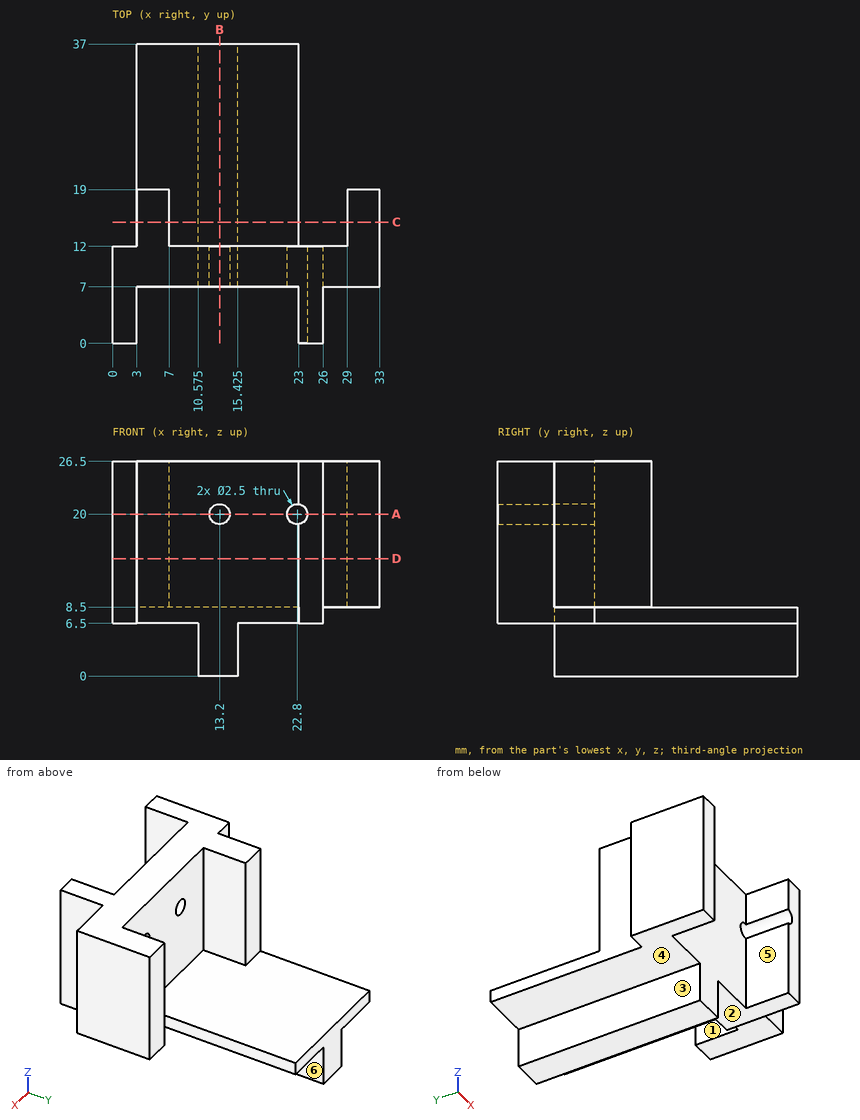
The drawing under review shows one solid part. Ordinate dimensions are in mm from its lowest x, y, z. A direction names the side the tool comes from. Coordinates: 2 decimals unless noted, no trailing zeros. Order: outer loops, then holes, each group sorted by start corner. A loop starts at its lowest first (then second) coordinate and runs counter-clockwise, first axis right, second up. Notation, with made-up numbers: (4, 5.25) -> (31, 5.25) arc R21 ccw to (31, 18.25) -> close; hole circle Ø10 at (-10, -31). An arc over 180 degrees is marked (long way). Answer in a Markdown table with one row per item. Add a question column.
Item 1: We need section B-B on x = 13.2. Write out the cut boundary in (y, z), plus the area to 4 significant figures.
Item 2: We need section D-D on z = 14.5. Write out the cut boundary in (x, y).
Item 3: Mouldability with a two-part tool opening along X and no side actions: class the marked faces 4, 5 and 6 as +X half, -X half, draft (parallel to the pull), parting line (faces both ways), or undercut.
Item 4: Clearance check with flat-ended pins moving along their axes: pin 1 (3 mm diameter, centred on x = 13.2, z = 20, fed in from -Y); pin 2 (3 mm diameter, centred on x = 7.5, y = 14, fed in from -Z); pin 3 (3 mm diameter, centred on x = 30.5, z = 17, fed in from +Y). State where each tip first meets the part, or that it passes through.
Item 5: To check wall thickness, follow probe 1 along X at (y, z) = (8.5, 20); probe 2 along X at (y, z) = (13.5, 24.5); probe 3 along X at (y, z) = (3.5, 16.75). State the ranges of each line that lie inside material, in increasing order.
Item 6: We need section A-A on z = 20. Write out the cut boundary in (x, y).
Item 7: We need section C-C on y = 15. Write out the cut boundary in (x, z) (3 decimals).
Item 8: Machinability: for the marked faces 1, 2 and 3, which of the approach directions +Z, -Z, +X, -X, +Y, -Y give a long, thin tool a straight path to every point of the face, cutting with its end or side? Answer none if there is none.
Final values:
| question | item | result |
|---|---|---|
| 1 | outline | (7, 0) -> (37, 0) -> (37, 8.5) -> (12, 8.5) -> (12, 18.75) -> (7, 18.75) -> close; (7, 21.25) -> (12, 21.25) -> (12, 26.5) -> (7, 26.5) -> close |
| 1 | area | 332.5 mm2 |
| 2 | outline | (0, 0) -> (3, 0) -> (3, 7) -> (23, 7) -> (23, 0) -> (26, 0) -> (26, 7) -> (33, 7) -> (33, 19) -> (29, 19) -> (29, 12) -> (7, 12) -> (7, 19) -> (3, 19) -> (3, 12) -> (0, 12) -> close |
| 3 | face 4 | draft |
| 3 | face 5 | undercut |
| 3 | face 6 | +X half |
| 4 | pin 1 | stops at y = 7 |
| 4 | pin 2 | stops at z = 6.5 |
| 4 | pin 3 | stops at y = 19 |
| 5 | probe 1 | x = 0 to 11.95, 14.45 to 21.55, 24.05 to 33 |
| 5 | probe 2 | x = 3 to 7, 29 to 33 |
| 5 | probe 3 | x = 0 to 3, 23 to 26 |
| 6 | outline | (0, 0) -> (3, 0) -> (3, 7) -> (11.95, 7) -> (11.95, 12) -> (7, 12) -> (7, 19) -> (3, 19) -> (3, 12) -> (0, 12) -> close; (14.45, 7) -> (21.55, 7) -> (21.55, 12) -> (14.45, 12) -> close; (24.05, 0) -> (26, 0) -> (26, 7) -> (33, 7) -> (33, 19) -> (29, 19) -> (29, 12) -> (24.05, 12) -> close |
| 7 | outline | (3, 6.5) -> (10.575, 6.5) -> (10.575, 0) -> (15.425, 0) -> (15.425, 6.5) -> (23, 6.5) -> (23, 8.5) -> (7, 8.5) -> (7, 26.5) -> (3, 26.5) -> close; (29, 8.5) -> (33, 8.5) -> (33, 26.5) -> (29, 26.5) -> close |
| 8 | face 1 | +Z, -Z, +Y |
| 8 | face 2 | -Z, +X, +Y, -Y |
| 8 | face 3 | -Z, -X, +Y, -Y |
